Part model, mm, in its own coordinate system. A direction names the side the tool comes from. Coordinates: 2 decimals unless noted, no trailing zeros. Write each loop counter-clockwise with the first axis right and the second up, starting at its lowest first coordinate (ties: lowest second). Pieces come first, ordered by that corner, then holes. Notation, with made-up numbers: (14, 67.25) - (42, 67.25) arc R9 cw to (42, 77.25) - close; hole circle Ø1 at (63, 3.25). An arc over 180 degrees is marked (long way). Use a Markdown table: item, result.
```python
from build123d import *

# Parameters (mm, degrees)
SKETCH_R        = 1.6
SKETCH_W        = 81.5
SKETCH_H        = 81.5
PAD_DEPTH       = 90
POCKET_DEPTH    = 120.001
SKETCH002_R     = 1.6
PAD001_DEPTH    = 4
POCKET001_DEPTH = 30
CHAMFER_SIZE    = 12.5
SKETCH005_W     = 13.5
SKETCH005_H     = 20
POCKET002_DEPTH = 90.001
SKETCH006_W     = 13.5
SKETCH006_H     = 24
POCKET003_DEPTH = 1
CHAMFER001_SIZE = 1.95
POCKET004_DEPTH = 15
FILLET_R        = 3


with BuildPart() as part:
    # Sketch → Pad (new body)
    with BuildSketch(Plane.XY):
        Polygon((-60, -48.5), (60, -48.5), (60, 48.5), (60, 83.5), (-60, 83.5), (-60, 48.5), align=None)
        with Locations((-53.75, 66)):
            Circle(SKETCH_R, mode=Mode.SUBTRACT)
        with Locations((-13.75, 66)):
            Circle(SKETCH_R, mode=Mode.SUBTRACT)
        with Locations((13.75, 66)):
            Circle(SKETCH_R, mode=Mode.SUBTRACT)
        with Locations((53.75, 66)):
            Circle(SKETCH_R, mode=Mode.SUBTRACT)
        Rectangle(SKETCH_W, SKETCH_H, mode=Mode.SUBTRACT)
        Polygon((-50.25, 53.5), (-17.25, 53.5), (-17.25, 71.5), (-24.25, 78.5), (-43.25, 78.5), (-50.25, 71.5), align=None, mode=Mode.SUBTRACT)
        Polygon((19.75, 56), (47.75, 56), (47.75, 71), (42.75, 76), (24.75, 76), (19.75, 71), align=None, mode=Mode.SUBTRACT)
    extrude(amount=PAD_DEPTH)

    # Sketch001 (on Face26 of Pad) → Pocket (cut, through all)
    with BuildSketch(Plane.YZ.offset(60)):
        with BuildLine():
            ThreePointArc((-40.7, 58), (-43, 60.3), (-45.3, 58))
            Line((-45.3, 58), (-48.5, 58))
            Line((-48.5, 0), (-48.5, 58))
            Line((-48.5, 0), (48.5, -0.061623))
            Line((48.5, -0.061623), (48.5, 58))
            Line((48.5, 58), (45.3, 58))
            ThreePointArc((45.3, 58), (43, 60.3), (40.7, 58))
            Line((30.966667, 58), (40.7, 58))
            ThreePointArc((30.966667, 58), (28.666667, 60.3), (26.366667, 58))
            Line((16.633333, 58), (26.366667, 58))
            ThreePointArc((16.633333, 58), (14.333333, 60.3), (12.033333, 58))
            Line((2.3, 58), (12.033333, 58))
            ThreePointArc((2.3, 58), (0, 60.3), (-2.3, 58))
            Line((-12.033333, 58), (-2.3, 58))
            ThreePointArc((-12.033333, 58), (-14.333333, 60.3), (-16.633333, 58))
            Line((-26.366667, 58), (-16.633333, 58))
            ThreePointArc((-26.366667, 58), (-28.666667, 60.3), (-30.966667, 58))
            Line((-40.7, 58), (-30.966667, 58))
        make_face()
    extrude(amount=-POCKET_DEPTH, mode=Mode.SUBTRACT)

    # Sketch002 (on Face24 of Pad) → Pad001 (join)
    with BuildSketch(Plane.XY.offset(90)):
        Polygon((-40.75, -40.75), (-40.75, -26.75), (-26.75, -40.75), align=None)
        with Locations((-36, -36)):
            Circle(SKETCH002_R, mode=Mode.SUBTRACT)
        Polygon((40.75, -40.75), (26.75, -40.75), (40.75, -26.75), align=None)
        with Locations((36, -36)):
            Circle(SKETCH002_R, mode=Mode.SUBTRACT)
        Polygon((40.75, 40.75), (40.75, 26.75), (26.75, 40.75), align=None)
        with Locations((36, 36)):
            Circle(SKETCH002_R, mode=Mode.SUBTRACT)
        Polygon((-40.75, 40.75), (-26.75, 40.75), (-40.75, 26.75), align=None)
        with Locations((-36, 36)):
            Circle(SKETCH002_R, mode=Mode.SUBTRACT)
    extrude(amount=-PAD001_DEPTH)

    # Sketch004 (on Face7 of Pad001) → Pocket001 (cut)
    with BuildSketch(Plane(origin=(0, 0, 0), x_dir=(1, 0, 0), z_dir=(0, 0, -1))):
        Polygon((-17.25, -53.5), (19.75, -56), (47.75, -56), (47.75, -71), (42.75, -76), (24.75, -76), (-24.25, -78.5), (-43.25, -78.5), (-50.25, -71.5), (-50.25, -53.5), align=None)
    extrude(amount=-POCKET001_DEPTH, mode=Mode.SUBTRACT)

    # Chamfer
    chamfer_edges = [part.edges().sort_by_distance(p)[0] for p in [
        (60, 83.5, 45),
        (-60, 83.5, 45),
    ]]
    chamfer(chamfer_edges, length=CHAMFER_SIZE)

    # Sketch005 → Pocket002 (cut, through all)
    with BuildSketch(Plane.XY.offset(90)):
        with Locations((0, 66)):
            Rectangle(SKETCH005_W, SKETCH005_H)
    extrude(amount=-POCKET002_DEPTH, mode=Mode.SUBTRACT)

    # Sketch006 (on Face8 of Pocket002) → Pocket003 (cut, symmetric)
    with BuildSketch(Plane.XY.offset(86)):
        with Locations((0, 66)):
            Rectangle(SKETCH006_W, SKETCH006_H)
    extrude(amount=POCKET003_DEPTH, both=True, mode=Mode.SUBTRACT)

    # Chamfer001
    chamfer001_edges = [part.edges().sort_by_distance(p)[0] for p in [
        (0, 76, 87),
        (0, 76, 85),
        (0, 56, 87),
        (0, 56, 85),
    ]]
    chamfer(chamfer001_edges, length=CHAMFER001_SIZE)

    # Sketch007 (on Face33 of Chamfer001) → Pocket004 (cut)
    with BuildSketch(Plane.XZ.offset(-40.75)):
        with BuildLine():
            ThreePointArc((-27, 71), (-30, 74), (-33, 71))
            Line((-33, 71), (-33, 65))
            ThreePointArc((-33, 65), (-30, 62), (-27, 65))
            Line((-27, 71), (-27, 65))
        make_face()
    extrude(amount=-POCKET004_DEPTH, mode=Mode.SUBTRACT)

    # Fillet
    fillet_edges = [part.edges().sort_by_distance(p)[0] for p in [
        (-30, 53.5, 62),
        (-33, 40.75, 68),
    ]]
    fillet(fillet_edges, radius=FILLET_R)


solid = part.part
```
Item 1: Drop a flat-ended pin along its axis: P1, Ø8, axis at x = 48.5, y = -34, coming from the -Z side. Give the stop position or say it passes through.
From the geometry:
| item | result |
|---|---|
| P1 | z = 58 |
Item 2: Two-plate mould, pull along Y, no slides. Class faces 5 (the face through (34.73, 35.03, 88.03)), 6 (the face through (-50, -36, 58)): pulls with the +Y half, pulls with the -Y half, needs draft (parallel to the pull), parting line crosses it, or undercut.
From the geometry:
| item | result |
|---|---|
| face 5 | undercut |
| face 6 | needs draft |
Item 3: Which spindle directions (+Z, -Z, +X, -X, +Y, -Y) get a long thin tool onto all of the face, cutting with end or side? Do faces 1 (the face through (50.5, -14.3, 60.3)), 2 (the face through (-33.8, -33.7, 88)), 3 (the face through (0.991, 54.732, 14.79)), 4 (the face through (-50, -22, 58)). Say none if no direction does.
From the geometry:
| item | result |
|---|---|
| face 1 | -Z, +X, -X |
| face 2 | +Z, -Z |
| face 3 | -Z |
| face 4 | -Z, +X, -X, -Y |
Item 4: Band-saw the part on C-C, the plane z = 26.5. Give the cut face in (x, y).
From the geometry:
| item | result |
|---|---|
| outline | (-60, 48.5) - (60, 48.5) - (60, 71) - (47.5, 83.5) - (-47.5, 83.5) - (-60, 71) - close; hole circle Ø3.2 at (-53.75, 66); hole (-50.25, 53.5) - (-17.25, 53.5) - (19.75, 56) - (47.75, 56) - (47.75, 71) - (42.75, 76) - (24.75, 76) - (-24.25, 78.5) - (-43.25, 78.5) - (-50.25, 71.5) - close; hole circle Ø3.2 at (53.75, 66) |
Item 5: Band-saw the part on A-A, the plane y = 20.5. Give the cut face in (x, z), then the cut area to 3 significant figures.
From the geometry:
| item | result |
|---|---|
| outline | (-60, 58) - (-40.75, 58) - (-40.75, 90) - (-60, 90) - close; (40.75, 58) - (60, 58) - (60, 90) - (40.75, 90) - close |
| area | 1,230 mm^2 |
Item 6: Band-saw the part on D-D, the plane y = 62. Give the cut face in (x, z).
From the geometry:
| item | result |
|---|---|
| outline | (-60, 0) - (-50.25, 0) - (-50.25, 90) - (-60, 90) - close; (-17.25, 30) - (-6.75, 30) - (-6.75, 90) - (-17.25, 90) - close; (6.75, 30) - (19.75, 30) - (19.75, 90) - (6.75, 90) - close; (47.75, 0) - (60, 0) - (60, 90) - (47.75, 90) - close |
Item 7: Band-saw the part on B-B, the plane x = -53.75. Give the cut face in (y, z).
From the geometry:
| item | result |
|---|---|
| outline | (-48.5, 58) - (-45.3, 58) arc R2.3 cw to (-40.7, 58) - (-30.97, 58) arc R2.3 cw to (-26.37, 58) - (-16.63, 58) arc R2.3 cw to (-12.03, 58) - (-2.3, 58) arc R2.3 cw to (2.3, 58) - (12.03, 58) arc R2.3 cw to (16.63, 58) - (26.37, 58) arc R2.3 cw to (30.97, 58) - (40.7, 58) arc R2.3 cw to (45.3, 58) - (48.5, 58) - (48.5, 0) - (64.4, 0) - (64.4, 90) - (-48.5, 90) - close; (67.6, 0) - (77.25, 0) - (77.25, 90) - (67.6, 90) - close |
Item 8: Drill centre lines: probe 1 along X at (y, z) = (62, 70); probe 2 along X at (y, z) = (-1, 61); probe 3 along Y at (x, z) = (22, 76.5). Where is each one in solid material? Low to high.
From the geometry:
| item | result |
|---|---|
| probe 1 | -60 to -50.25, -17.25 to -6.75, 6.75 to 19.75, 47.75 to 60 |
| probe 2 | -60 to -40.75, 40.75 to 60 |
| probe 3 | -48.5 to -40.75, 40.75 to 56, 73.25 to 83.5 |
